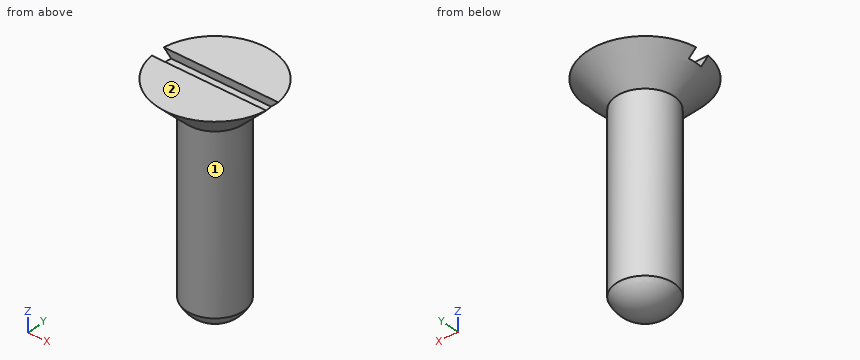
```python
from build123d import *

# Parameters (mm, degrees)
F2_W     = 10.128174
F2_H     = 1
F3_DEPTH = 0.5


with BuildPart() as f1:
    # F0 (on Front) → F1 (revolve)
    with BuildSketch(Plane.XZ):
        with BuildLine():
            Line((0, 14), (0, 0))
            Line((0, 0), (0, -1.251342))
            ThreePointArc((0, -1.251342), (1.181918, -0.916427), (2, 0))
            Line((2, 0), (2, 12))
            Line((2, 12), (4, 14))
            Line((4, 14), (0, 14))
        make_face()
    revolve(axis=Axis((0, 0, 7), (0, 0, 1)))

    # F2 (on face) → F3 (cut)
    with BuildSketch(Plane.XY.offset(14)):
        Rectangle(F2_W, F2_H)
    extrude(amount=-F3_DEPTH, mode=Mode.SUBTRACT)


solid = f1.part
```
Can you work these out from the model? Positions are in its coordinate system, mm. Face numbers are marked on the shaded views. A direction names the side the tool comes from. Coordinates: 2 decimals unless noted, no trailing zeros. Order: outer loops, then holes, each group sorted by start corner. A loop starts at its lowest first (then second) coordinate and runs counter-clockwise, first axis right, second up.
1. I need wall thicknesses on line 1 (Z direction, x = -2.75, y = 2.5); line 2 (Z direction, x = 2, y = -2.5); line 3 (Y direction, x = -1, z = 9.75). Which ranges of each line are inside material? Lowest first, please.
2. I'm going to push flat-ended pins straight in: pin 1 (1 mm diameter, centred on y = -0.5, z = 9.5, fed in from -X); pin 2 (2 mm diameter, centred on x = 0.5, y = -2, fed in from -Z); pin 3 (1.5 mm diameter, centred on x = -1, z = 8.5, fed in from -Y). Where does each tip first touch, or does it pass through?
3. For the marked faces 1 and 2, which set-ups out of +Z, -Z, +X, -X, +Y, -Y let a thin tool reach every point of the face, with its end or its side?
4. If we section it at A-A (z = 4): Please give me the cut outline in (x, y), then the cut area to 3 significant figures.
Entries:
1. line 1: z = 13.72 to 14
1. line 2: z = 13.2 to 14
1. line 3: y = -1.73 to 1.73
2. pin 1: stops at x = -2
2. pin 2: stops at z = -0.99
2. pin 3: stops at y = -1.98
3. face 1: -Z
3. face 2: +Z, +X, -X, +Y, -Y
4. outline: circle Ø4 at (0, 0)
4. area: 12.6 mm2
